```python
from build123d import *

# Parameters (mm, degrees)
BOSS_EXTRUDE1_DEPTH = 8
CUT_EXTRUDE1_DEPTH  = 17.492422502
CUT_EXTRUDE2_DEPTH  = 1.99
CUT_EXTRUDE4_REACH  = 23.541
SKETCH6_W           = 4
SKETCH6_H           = 8
SKETCH7_R           = 1.6
CUT_EXTRUDE5_DEPTH  = 22.540659229
CHAMFER1_SIZE       = 0.5


with BuildPart() as part:
    # Sketch1 → Boss-Extrude1 (new body)
    with BuildSketch(Plane.XY.offset(8)):
        with BuildLine():
            Line((8, 0), (8, 12))
            Line((8, 12), (-8, 12))
            Line((-8, 12), (-8, 0))
            ThreePointArc((-8, 0), (0, -8), (8, 0))
        make_face()
    extrude(amount=-BOSS_EXTRUDE1_DEPTH)

    # Sketch2 → Cut-Extrude1 (cut, through all)
    with BuildSketch(Plane(origin=(0, 0, 0), x_dir=(-1, 0, 0), z_dir=(0, 0, -1))):
        with BuildLine():
            Line((2.5, 12), (-2.5, 12))
            Line((-2.5, 12), (-2.5, 3.122498999))
            ThreePointArc((-2.5, 3.122498999), (0, 4), (2.5, 3.122498999))
            Line((2.5, 3.122498999), (2.5, 12))
        make_face()
    extrude(amount=-CUT_EXTRUDE1_DEPTH, mode=Mode.SUBTRACT)

    # Sketch3 → Cut-Extrude2 (cut)
    with BuildSketch(Plane.ZY.offset(8)):
        Polygon((5.674315, 4.100001352), (7.34863, 7), (5.674315, 9.899998648), (2.325685, 9.899998648), (0.65137, 7), (2.325685, 4.100001352), align=None)
    extrude(amount=-CUT_EXTRUDE2_DEPTH, mode=Mode.SUBTRACT)

    # Sketch5 → Cut-Extrude4 (cut, up to next)
    with BuildSketch(Plane(origin=(8, 0, 0), x_dir=(0, 0, -1), z_dir=(1, 0, 0)), mode=Mode.PRIVATE) as cut_extrude4_sk1:
        Polygon((-5.33035138, 6.111087627), (-5.13137085, 5.86862915), (-4.888912373, 5.66964862), (-4.612293492, 5.521792748), (-4.312144515, 5.430743551), (-4, 5.4), (-3.687855485, 5.430743551), (-3.387706508, 5.521792748), (-3.111087627, 5.66964862), (-2.86862915, 5.86862915), (-2.66964862, 6.111087627), (-2.521792748, 6.387706508), (-2.430743551, 6.687855485), (-2.4, 7), (-2.430743551, 7.312144515), (-2.521792748, 7.612293492), (-2.66964862, 7.888912373), (-2.86862915, 8.13137085), (-3.111087627, 8.33035138), (-3.387706508, 8.478207252), (-3.687855485, 8.569256449), (-4, 8.6), (-4.312144515, 8.569256449), (-4.612293492, 8.478207252), (-4.888912373, 8.33035138), (-5.13137085, 8.13137085), (-5.33035138, 7.888912373), (-5.478207252, 7.612293492), (-5.569256449, 7.312144515), (-5.6, 7), (-5.569256449, 6.687855485), (-5.478207252, 6.387706508), align=None)
    cut_extrude4_tool1 = extrude(cut_extrude4_sk1.sketch, amount=-CUT_EXTRUDE4_REACH, mode=Mode.PRIVATE) & part.part
    add(cut_extrude4_tool1.solids().sort_by_distance((8, 7, 4))[0], mode=Mode.SUBTRACT)

    # Sketch6 → Cut-Revolve1 (revolve, cut)
    with BuildSketch(Plane(origin=(0, 0, 0), x_dir=(1, 0, 0), z_dir=(0, 1, 0))):
        with Locations((2, -4)):
            Rectangle(SKETCH6_W, SKETCH6_H)
    revolve(axis=Axis((0, 0, 0), (0, 0, 1)), mode=Mode.SUBTRACT)

    # Sketch7 → Cut-Extrude5 (cut, through all)
    with BuildSketch(Plane(origin=(8, 0, 0), x_dir=(0, 0, -1), z_dir=(1, 0, 0))):
        with Locations(Location((-4, 7, 0), (0, 0, 270))):
            Circle(SKETCH7_R)
    extrude(amount=-CUT_EXTRUDE5_DEPTH, mode=Mode.SUBTRACT)

    # Chamfer1
    chamfer1_edges = [part.edges().sort_by_distance(p)[0] for p in [
        (5.25, 12, 0),
        (-8, 6, 0),
        (0, -4, 0),
        (-5.25, 12, 0),
        (-2.5, 7.5612495, 0),
        (2.5, 7.5612495, 0),
        (0, -8, 0),
        (8, 6, 0),
    ]]
    chamfer(chamfer1_edges, length=CHAMFER1_SIZE)


solid = part.part
```
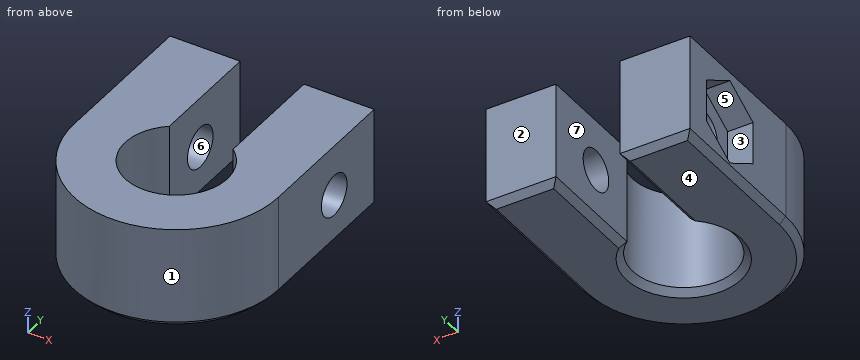
Here's how the part is built. I have some questions about the finished solid (model axes, mm). Face numbers are marked on the shaded views. A direction names the side the tool comes from. Round coordinates to 2 decimals unless told otherwise and drop trailing zeros. Order: outer loops, then holes, each group sorted by start corner. A loop starts at its lowest first (then second) coordinate and runs counter-clockwise, first axis right, second up. Notation, with made-up numbers: M 14,-36.5 L 66,-36.5 A18 cw 66,-11.5 Z; hole C -14,68.5 d1. An arc over 180 degrees is marked long. Answer in a Markdown table with one row per item.
Item 1: I'm going to push flat-ended pins straight in: pin 1 (3 mm diameter, centred on y = 7.5, z = 4.5, fed in from -X); pin 2 (2 mm diameter, centred on y = -5, z = 4.5, fed in from +X); pin 3 (1 mm diameter, centred on x = -6.5, z = 4, fed in from -Y). Where does each tip first touch, or does it pass through?
A:
| item | result |
|---|---|
| pin 1 | stops at x = -6.01 |
| pin 2 | stops at x = 6.93 |
| pin 3 | stops at y = -5.29 |
Item 2: If I drill on L1, parallel to X at y = 8, z = 2.25; L2, parallel to X at y = 0, z = 4; L3, parallel to Z at x = -3.3, y = 7, over which ranges is the centre line in solid material (lowest first)? Write a range as from..to.
A:
| item | result |
|---|---|
| L1 | x = -6.01..-2.5, 2.5..8 |
| L2 | x = -8..-4, 4..8 |
| L3 | z = 0..2.4, 5.6..8 |
Item 3: For the marked faces 5, 6 and 7, which set-ups out of +Z, -Z, +X, -X, +Y, -Y let a thin tool reach every point of the face, with its end or its side?
A:
| item | result |
|---|---|
| face 5 | -X |
| face 6 | +X, -X |
| face 7 | +Z, -Z, +Y |
Item 4: Thinking about a two-plate mould opening in Y: for the marked faces 1, 2, 3 and 4, which applies, +Y half, -Y half, draft (parallel to the pull), parting line (faces both ways), or undercut?
A:
| item | result |
|---|---|
| face 1 | -Y half |
| face 2 | +Y half |
| face 3 | undercut |
| face 4 | draft |
Item 5: Imagine slicing it at B-B, the plane y = 9. Write out the boundary of the cut face in (x, z), and give its area (3 significant figures).
A:
| item | result |
|---|---|
| outline | M -8,0.5 L -7.5,0 L -3,0 L -2.5,0.5 L -2.5,8 L -8,8 L -8,6.19 L -6.01,6.19 L -6.01,1.81 L -8,1.81 Z; M 2.5,0.5 L 3,0 L 7.5,0 L 8,0.5 L 8,8 L 2.5,8 Z |
| area | 78.8 mm2 |
Item 6: Imagine slicing it at D-D, the plane z = 1.5. Write out the boundary of the cut face in (x, y).
A:
| item | result |
|---|---|
| outline | M -8,0 A8 ccw 8,0 L 8,12 L 2.5,12 L 2.5,3.12 A4 cw long -2.5,3.12 L -2.5,12 L -8,12 L -8,8.47 L -6.01,8.47 L -6.01,5.53 L -8,5.53 Z |
Item 7: Imagine slicing it at A-A, the plane z = 4. Write out the boundary of the cut face in (x, y), and give its area (4 significant figures).
A:
| item | result |
|---|---|
| outline | M -8,0 A8 ccw 8,0 L 8,5.4 L 2.5,5.4 L 2.5,3.12 A4 cw long -2.5,3.12 L -2.5,5.4 L -6.01,5.4 L -6.01,4.1 L -8,4.1 Z; M -8,9.9 L -6.01,9.9 L -6.01,8.6 L -2.5,8.6 L -2.5,12 L -8,12 Z; M 2.5,8.6 L 8,8.6 L 8,12 L 2.5,12 Z |
| area | 160.5 mm2 |
Item 8: Imagine slicing it at C-C, the plane x = 0. Write out the boundary of the cut face in (y, z).
A:
| item | result |
|---|---|
| outline | M -8,0.5 L -7.5,0 L -4.5,0 L -4,0.5 L -4,8 L -8,8 Z |
